```python
from build123d import *

# Parameters (mm, degrees)
F1_DEPTH = 300


with BuildPart() as f1:
    # F0 (on Front) → F1 (new body)
    with BuildSketch(Plane.XZ):
        with BuildLine():
            Line((-33.991796, -5.594154), (-33.991796, -10.594154))
            Line((-33.991796, -10.594154), (6.008204, -10.594154))
            Line((6.008204, -10.594154), (6.008204, -5.594154))
            Line((6.008204, -5.594154), (-4.741796, -5.594154))
            Line((-4.741796, -5.594154), (-4.741796, 1.051143))
            Line((-4.741796, 1.051143), (-9.991796, 1.051143))
            Line((-9.991796, 1.051143), (-9.991796, 7.205846))
            Line((-9.991796, 7.205846), (-10.504677, 7.205846))
            ThreePointArc((-10.504677, 7.205846), (-13.991796, 22.405846), (-17.478915, 7.205846))
            Line((-17.478915, 7.205846), (-17.991796, 7.205846))
            Line((-17.991796, 7.205846), (-17.991796, 1.051143))
            Line((-17.991796, 1.051143), (-23.241796, 1.051143))
            Line((-23.241796, 1.051143), (-23.241796, -5.594154))
            Line((-23.241796, -5.594154), (-33.991796, -5.594154))
        make_face()
    extrude(amount=F1_DEPTH)


solid = f1.part
```
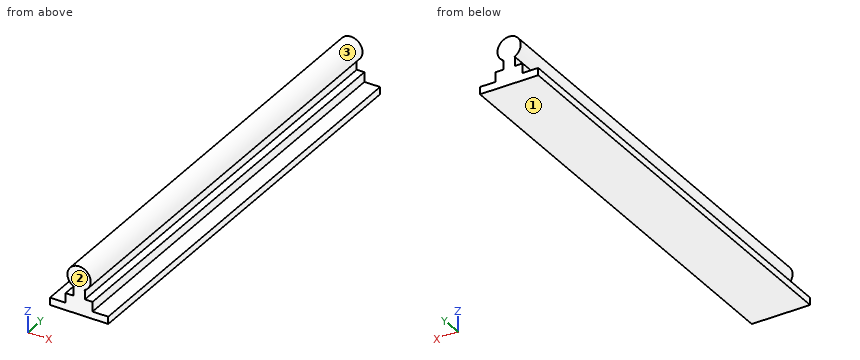
Geometry: final body of the model. Coordinates: model frame, mm. Face numbers are marked on the shaded views. Round coordinates to 2 decimals unless told otherwise and drop trailing zeros. Loops run counter-clockwise (first coordinate to the right, second up) from the corner with the lowest first, then second, coordinate; pieces in that order, holes last.
Item 1: Section C-C, the plane z = 11. Output: boundary loops of the cut face in (x, y), plus the area to 3 significant figures.
Checked values:
outline: (-21.23, -300) - (-6.75, -300) - (-6.75, 0) - (-21.23, 0) - close
area: 4,340 mm2
Item 2: Contact query for flat-ended pins moving along their axis: P1, Ø4, axis at y = -262.5, z = 9.5, coming from the +X side; P2, Ø5, axis at y = -218, z = 3, coming from the +X side; P3, Ø12, axis at x = 1.5, y = -224.5, coming from the +Z side. Output: stop coordinate, or through.
Checked values:
P1: stops at x = -6.54
P2: stops at x = -4.74
P3: stops at z = -5.59
Item 3: Section B-B, the plane x = 2.5. Output: boundary loops of the cut face in (y, z), plus the area to 3 significant figures.
Checked values:
outline: (-300, -10.59) - (0, -10.59) - (0, -5.59) - (-300, -5.59) - close
area: 1,500 mm2
Item 4: Mould query, pull axis Z, two halves, no side actions, for the marked faces 1, 2 and 3. Classes: released by +Z, released by -Z, zero draft, split by the parting line, or undercut.
Checked values:
face 1: released by -Z
face 2: zero draft
face 3: undercut
Item 5: Section A-A, the plane y = -43. Output: boundary loops of the cut face in (x, z).
Checked values:
outline: (-33.99, -10.59) - (6.01, -10.59) - (6.01, -5.59) - (-4.74, -5.59) - (-4.74, 1.05) - (-9.99, 1.05) - (-9.99, 7.21) - (-10.5, 7.21) arc R8 ccw (long way) to (-17.48, 7.21) - (-17.99, 7.21) - (-17.99, 1.05) - (-23.24, 1.05) - (-23.24, -5.59) - (-33.99, -5.59) - close
Item 6: Line query: L1, parallel to X at y = -163.5, z = -4.5; L2, parallel to X at y = -78, z = 14; L3, parallel to Z at x = -5, y = -30.5. Output: solid intervals per line, ascending.
Checked values:
L1: x = -23.24 to -4.74
L2: x = -21.98 to -6
L3: z = -10.59 to 1.05
